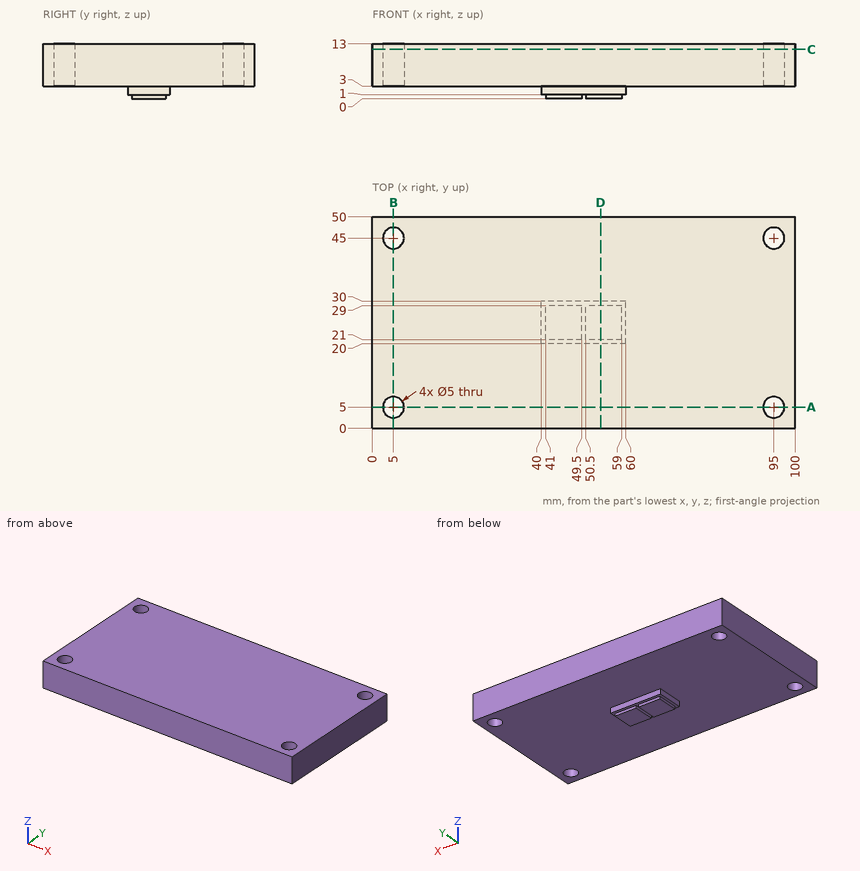
Can you work these out from the drawing? Everything is in mm from the part's minimum corner. Give positions to 0.01 mm unless a question says otherwise; leave off trailing zeros. Order: outer loops, then holes, each group sorted by start corner. A loop starts at its lowest first (then second) coordinate and runs counter-clockwise, first axis right, second up. Notation, with made-up numbers: M -9.75,-29.75 L 8.25,-29.75 A29 ccw 8.25,9.25 Z; hole C 80.5,-39 d6. An arc over 180 degrees is marked long. Use a Markdown table: item, result. Add a question column.
1. For pin 1 Ø0.8 at (y, z) = (23.5, 0.5) entering from +X; pin 2 Ø0.8 at (x, z) = (55.5, 0.5) entering from +Y; pin 3 Ø4.5 at (x, y) = (5, 45) entering from +Z; pin 4 Ø1.6 at (y, z) = (24.5, 2) entering from -X, each with a flat end and sliding along its axis, tell me the tip position at first contact or that it passes through.
2. Suppose I cut it at A-A (y = 5). List the corners of the cut face in (x, z) for me.
3. I need wall thicknesses on probe 1 along Y at (x, z) = (95, 10.5); probe 2 along X at (y, z) = (46, 10.75); probe 3 along Z at (x, y) = (76.5, 20). Which ranges of each line are inside material? Lowest first, please. Write a range as from..to.
4. Suppose I cut it at B-B (x = 5). List the corners of the cut face in (y, z) for me.
5. Suppose I cut it at C-C (z = 11.75). List the corners of the cut face in (x, y) for me.
6. Suppose I cut it at D-D (x = 54). List the corners of the cut face in (y, z) for me, and give its area (3 significant figures).
Results list:
| question | item | result |
|---|---|---|
| 1 | pin 1 | stops at x = 59 |
| 1 | pin 2 | stops at y = 29 |
| 1 | pin 3 | passes through |
| 1 | pin 4 | stops at x = 40 |
| 2 | outline | M 0,3 L 2.5,3 L 2.5,13 L 0,13 Z; M 7.5,3 L 92.5,3 L 92.5,13 L 7.5,13 Z; M 97.5,3 L 100,3 L 100,13 L 97.5,13 Z |
| 3 | probe 1 | y = 0..2.5, 7.5..42.5, 47.5..50 |
| 3 | probe 2 | x = 0..2.71, 7.29..92.71, 97.29..100 |
| 3 | probe 3 | z = 3..13 |
| 4 | outline | M 0,3 L 2.5,3 L 2.5,13 L 0,13 Z; M 7.5,3 L 42.5,3 L 42.5,13 L 7.5,13 Z; M 47.5,3 L 50,3 L 50,13 L 47.5,13 Z |
| 5 | outline | M 0,0 L 100,0 L 100,50 L 0,50 Z; hole C 5,5 d5; hole C 5,45 d5; hole C 95,5 d5; hole C 95,45 d5 |
| 6 | outline | M 0,3 L 20,3 L 20,1 L 21,1 L 21,0 L 29,0 L 29,1 L 30,1 L 30,3 L 50,3 L 50,13 L 0,13 Z |
| 6 | area | 528 mm² |
